```python
from build123d import *

# Parameters (mm, degrees)
F1_DEPTH = 3
F2_R     = 17.5
F2_R_2   = 13
F2_R_3   = 2
F2_W     = 22
F2_H     = 50
F2_W_2   = 50
F2_H_2   = 22
F3_DEPTH = 3
F4_R     = 2.5
F5_DEPTH = 3
F6_R     = 3.25
F7_DEPTH = 3
F8_R     = 3.25
F9_DEPTH = 3
F10_R    = 5


# Not quite as in the source:
# - a feature names something its author has since deleted; it is built from what else it names


with BuildPart() as f1:
    # F0 (on Front) → F1 (new body)
    with BuildSketch(Plane.XZ):
        Polygon((90, -75), (90, 75), (-90, 75), (-90, -75), (-50, -75), (-50, -120), (90, -120), align=None)
    extrude(amount=F1_DEPTH)

    # F2 (on face) → F3 (cut, through all)
    with BuildSketch(Plane.XZ.offset(3)):
        with Locations((-65, 40)):
            Circle(F2_R)
        with Locations((-65, -40)):
            Circle(F2_R_2)
        with BuildLine():
            ThreePointArc((-50.3238814883, 57.7090808748), (-50.2202795796, 54.7797204204), (-47.2909191252, 54.6761185117))
            ThreePointArc((-47.2909191252, 54.6761185117), (-48.7365440327, 56.2634559673), (-50.3238814883, 57.7090808748))
        make_face()
        with BuildLine():
            ThreePointArc((-50.3238814883, 57.7090808748), (-48.7365440327, 56.2634559673), (-47.2909191252, 54.6761185117))
            ThreePointArc((-47.2909191252, 54.6761185117), (-46.7439805879, 55.4075382028), (-46.55, 56.3))
            ThreePointArc((-46.55, 56.3), (-47.9479511984, 58.3141803792), (-50.3238814883, 57.7090808748))
        make_face()
        with BuildLine():
            ThreePointArc((-82.7125051724, 25.3280144317), (-82.7202795796, 22.2797204204), (-79.6719855683, 22.2874948276))
            ThreePointArc((-79.6719855683, 22.2874948276), (-81.2634559673, 23.7365440327), (-82.7125051724, 25.3280144317))
        make_face()
        with BuildLine():
            ThreePointArc((-82.7125051724, 25.3280144317), (-81.2634559673, 23.7365440327), (-79.6719855683, 22.2874948276))
            ThreePointArc((-79.6719855683, 22.2874948276), (-79.2115670708, 22.9822992687), (-79.05, 23.8))
            ThreePointArc((-79.05, 23.8), (-80.3721673239, 25.7842361403), (-82.7125051724, 25.3280144317))
        make_face()
        with Locations((-25, -40)):
            Circle(F2_R_3)
        with Locations((25, -40)):
            Circle(F2_R_3)
        with Locations((64, -40)):
            Circle(F2_R_2)
        with Locations((61, 30)):
            Rectangle(F2_W, F2_H)
        with Locations((5, 40)):
            Rectangle(F2_W_2, F2_H_2)
    extrude(amount=-F3_DEPTH, mode=Mode.SUBTRACT)

    # F4 (on face) → F5 (cut, through all)
    with BuildSketch(Plane.XZ.offset(3)):
        with Locations((-85, 70)):
            Circle(F4_R)
        with Locations((85, 70)):
            Circle(F4_R)
        with Locations((20, -115)):
            Circle(F4_R)
        with Locations((-85, -70)):
            Circle(F4_R)
    extrude(amount=-F5_DEPTH, mode=Mode.SUBTRACT)

    # F6 (on face) → F7 (cut, through all)
    with BuildSketch(Plane.XZ.offset(3)):
        with Locations((-32, -89.5)):
            Circle(F6_R)
        with Locations((-16, -89.5)):
            Circle(F6_R)
        with Locations((0, -89.5)):
            Circle(F6_R)
        with Locations((40, -89.5)):
            Circle(F6_R)
        with Locations((56, -89.5)):
            Circle(F6_R)
        with Locations((72, -89.5)):
            Circle(F6_R)
        with Locations((72, -105.5)):
            Circle(F6_R)
        with Locations((56, -105.5)):
            Circle(F6_R)
        with Locations((40, -105.5)):
            Circle(F6_R)
        with Locations((-32, -105.5)):
            Circle(F6_R)
        with Locations((-16, -105.5)):
            Circle(F6_R)
        with Locations((0, -105.5)):
            Circle(F6_R)
    extrude(amount=-F7_DEPTH, mode=Mode.SUBTRACT)

    # F8 (on face) → F9 (cut, through all)
    with BuildSketch(Plane.XZ.offset(3)):
        with Locations((-10, 56)):
            Circle(F8_R)
        with Locations((20, 56)):
            Circle(F8_R)
        with Locations((77, 15)):
            Circle(F8_R)
        with Locations((77, 45)):
            Circle(F8_R)
    extrude(amount=-F9_DEPTH, mode=Mode.SUBTRACT)

    # F10
    f10_edges = [f1.edges().sort_by_distance(p)[0] for p in [
        (90, -1.5, 75),
        (-90, -1.5, 75),
        (-90, -1.5, -75),
        (-50, -1.5, -120),
        (90, -1.5, -120),
    ]]
    fillet(f10_edges, radius=F10_R)


solid = f1.part
```
Read the model definition and answer for the solid it produces. Units are mm, in the model's axes. Give positions to 0.01 mm unless a question says otherwise; leave off trailing zeros. Write each loop counter-clockwise with the first axis right and the second up, starting at its lowest first coordinate (ties: lowest second). Pieces come first, ordered by that corner, then holes. Notation, with made-up numbers: (87.5, 61.5) -> (113.5, 61.5) arc R19 ccw to (113.5, 96.5) -> close; hole circle Ø11 at (16, -20). An arc over 180 degrees is marked (long way). Answer in a Markdown table with one row per item.
1) Straight lines are drawn through the part: line 1 (Z direction, x = -13, y = -2.1); line 2 (Z direction, x = -77, y = -2.2); line 3 (Z direction, x = -16, y = -1.6). For each, find the intervals that lie inside material, in ascending order. Write a range as [from, to].
Results list:
| item | result |
|---|---|
| line 1 | [-120, -106.75], [-104.25, -90.75], [-88.25, 29], [51, 54.75], [57.25, 75] |
| line 2 | [-75, -45], [-35, 27.26], [52.74, 75] |
| line 3 | [-120, -108.75], [-102.25, -92.75], [-86.25, 29], [51, 75] |
2) Section C-C on x = 56.5 is taken. Give the vertices of the cut face in (y, z).
Results list:
| item | result |
|---|---|
| outline | (-3, -120) -> (0, -120) -> (0, -108.71) -> (-3, -108.71) -> close; (-3, -102.29) -> (0, -102.29) -> (0, -92.71) -> (-3, -92.71) -> close; (-3, -86.29) -> (0, -86.29) -> (0, -50.62) -> (-3, -50.62) -> close; (-3, -29.38) -> (0, -29.38) -> (0, 5) -> (-3, 5) -> close; (-3, 55) -> (0, 55) -> (0, 75) -> (-3, 75) -> close |
3) Section B-B on x = -16 is taken. Give the vertices of the cut face in (y, z), plus the area to 3 significant figures.
Results list:
| item | result |
|---|---|
| outline | (-3, -120) -> (0, -120) -> (0, -108.75) -> (-3, -108.75) -> close; (-3, -102.25) -> (0, -102.25) -> (0, -92.75) -> (-3, -92.75) -> close; (-3, -86.25) -> (0, -86.25) -> (0, 29) -> (-3, 29) -> close; (-3, 51) -> (0, 51) -> (0, 75) -> (-3, 75) -> close |
| area | 480 mm^2 |
4) Determine the mould class of faces 1 (the cylindrical face through (74.421, -1.521, 43.022)), 2 (the cylindrical face through (-88, -2, 74)), 3 (the cylindrical face through (89, -2, -118)) for opening direction Z: released by +Z, released by -Z, zero draft, split by the parting line, or undercut.
Results list:
| item | result |
|---|---|
| face 1 | undercut |
| face 2 | released by +Z |
| face 3 | released by -Z |
5) Section D-D on y = -2.55 is taken. Count the separate pieces of the cut face and the enclosed holes in it, plus the area to 3 significant figures.
Results list:
| item | result |
|---|---|
| separate pieces | 1 |
| enclosed holes | 29 |
| area | 28,400 mm^2 |
6) Section A-A on z = -105.5 is taken. Give the vertices of the cut face in (x, y), plus the area to 3 significant figures.
Results list:
| item | result |
|---|---|
| outline | (-50, -3) -> (-35.25, -3) -> (-35.25, 0) -> (-50, 0) -> close; (-28.75, -3) -> (-19.25, -3) -> (-19.25, 0) -> (-28.75, 0) -> close; (-12.75, -3) -> (-3.25, -3) -> (-3.25, 0) -> (-12.75, 0) -> close; (3.25, -3) -> (36.75, -3) -> (36.75, 0) -> (3.25, 0) -> close; (43.25, -3) -> (52.75, -3) -> (52.75, 0) -> (43.25, 0) -> close; (59.25, -3) -> (68.75, -3) -> (68.75, 0) -> (59.25, 0) -> close; (75.25, -3) -> (90, -3) -> (90, 0) -> (75.25, 0) -> close |
| area | 303 mm^2 |
